Build history of the part. All positions in model axes, mm. Give positions to 0.01 mm unless a question says otherwise; leave off trailing zeros. Order: outer loops, then holes, each group sorted by start corner. A loop starts at its lowest first (then second) coordinate and runs counter-clockwise, first axis right, second up. Notation, with made-up numbers: M 50,-4.5 L 104,-4.5 A29 ccw 104,16.5 Z; hole C 78,65 d8. An arc over 180 degrees is marked long. Use CSV: the item, a comma, the result in double quotes. Start each with the question number.
Item 1: Band-saw the part on B-B on x = 102. Write the cut outline in (y, z), plus the area to 3 significant figures.
Item 2: Wall check: line 1 along Z through (x, y) = (73, -17.25); line 2 along X through (y, z) = (-14.25, -103); line 3 along X through (y, z) = (-3.5, -19.5). Give the ranges that are in metal, low to high.
Item 3: Band-saw the part on A-A on y = -16.25. Give the number of separate pieces and of enclosed holes in the cut face, plus the area to 3 significant figures.
Item 4: Band-saw the part on D-D on x = -9. Write the cut outline in (y, z), plus the area to 3 significant figures.
Item 5: Two-plate mould, pull along Z, no slides. Class faces 1 (the flat face through (119.332, -12.522, 66.103)), 2 (the flat face through (162.666, -13, -65)): pulls with the +Z half, pulls with the -Z half, needs draft (parallel to the pull), parting line crosses it, or undercut.
Item 6: Band-saw the part on C-C on z = -166.5. Write the cut outline in (x, y).
from build123d import *

# Parameters (mm, degrees)
F0_W     = 189.734152
F0_H     = 298.390715
F1_DEPTH = 25.4


with BuildPart() as f1:
    # F0 (on Front) → F1 (new body)
    with BuildSketch(Plane.XZ):
        with Locations((67.798666, -63.308537)):
            Rectangle(F0_W, F0_H)
        Polygon((0, -58.81841), (-14.36841, -44.45), (-14.36841, 44.45), (0, 58.81841), (8.980256, 58.81841), (23.348666, 73.18682), (112.248666, 73.18682), (126.617076, 58.81841), (135.597332, 58.81841), (149.965742, 44.45), (149.965742, -44.45), (135.597332, -58.81841), (135.597332, -67.798666), (149.965742, -82.167076), (149.965742, -171.067076), (135.597332, -185.435486), (126.617076, -185.435486), (112.248666, -199.803895), (23.348666, -199.803895), (8.980256, -185.435486), (0, -185.435486), (-14.36841, -171.067076), (-14.36841, -82.167076), (0, -67.798666), align=None, mode=Mode.SUBTRACT)
        Polygon((14.36841, 44.45), (14.36841, -44.45), (0, -58.81841), (0, -67.798666), (4.490128, -63.308538), (18.858538, -48.940128), (116.738794, -48.940128), (131.107204, -63.308538), (135.597332, -67.798666), (135.597332, -58.81841), (121.228922, -44.45), (121.228922, 44.45), (135.597332, 58.81841), (126.617076, 58.81841), (112.248666, 44.45), (23.348666, 44.45), (8.980256, 58.81841), (0, 58.81841), align=None)
        Polygon((4.490128, -63.308538), (0, -67.798666), (14.36841, -82.167076), (14.36841, -171.067076), (0, -185.435486), (8.980256, -185.435486), (23.348666, -171.067076), (112.248666, -171.067076), (126.617076, -185.435486), (135.597332, -185.435486), (121.228922, -171.067076), (121.228922, -82.167076), (135.597332, -67.798666), (131.107204, -63.308538), (116.738794, -77.676948), (18.858538, -77.676948), align=None)
        Polygon((149.965742, 44.45), (135.597332, 58.81841), (121.228922, 44.45), (121.228922, -44.45), (135.597332, -58.81841), (149.965742, -44.45), align=None)
        Polygon((14.36841, -82.167076), (0, -67.798666), (-14.36841, -82.167076), (-14.36841, -171.067076), (0, -185.435486), (14.36841, -171.067076), align=None)
    extrude(amount=F1_DEPTH)


solid = f1.part
Model answer:
1,outline,"M -25.4,-212.5 L 0,-212.5 L 0,-199.8 L -25.4,-199.8 Z; M -25.4,-171.07 L 0,-171.07 L 0,-77.68 L -25.4,-77.68 Z; M -25.4,-48.94 L 0,-48.94 L 0,44.45 L -25.4,44.45 Z; M -25.4,73.19 L 0,73.19 L 0,85.89 L -25.4,85.89 Z"
1,area,"5,390 mm^2"
2,line 1,"z = -212.5 to -199.8, -171.07 to -77.68, -48.94 to 44.45, 73.19 to 85.89"
2,line 2,"x = -27.07 to 121.23, 149.97 to 162.67"
2,line 3,"x = -27.07 to -14.37, 14.37 to 162.67"
3,separate pieces,"1"
3,enclosed holes,"5"
3,area,"41,500 mm^2"
4,outline,"M -25.4,-212.5 L 0,-212.5 L 0,-49.82 L -25.4,-49.82 Z; M -25.4,49.82 L 0,49.82 L 0,85.89 L -25.4,85.89 Z"
4,area,"5,050 mm^2"
5,face 1,"undercut"
5,face 2,"needs draft"
6,outline,"M -27.07,-25.4 L 121.23,-25.4 L 121.23,0 L -27.07,0 Z; M 149.97,-25.4 L 162.67,-25.4 L 162.67,0 L 149.97,0 Z"
